CAD build for the part. Positions are in the model's coordinates, mm. A direction names the side the tool comes from. Round coordinates to 2 decimals unless told otherwise and drop trailing zeros. Order: outer loops, then holes, each group sorted by start corner. A loop starts at its lowest first (then second) coordinate and runs counter-clockwise, first axis right, second up. Notation, with made-up numbers: M -37,-32 L -2,-32 A11 ccw -2,-23 Z; hole C 38,-17 d6. An arc over 180 degrees is marked long. Answer as a JSON object with one key per item and string values.
```python
from build123d import *

# Parameters (mm, degrees)
EXTRUDE_1_DEPTH = 1.5
SKETCH_2_R      = 3
EXTRUDE_2_DEPTH = 7
EXTRUDE_START   = 3.5
EXTRUDE_3_DEPTH = 1.5
SKETCH_3_R      = 2.5
EXTRUDE_4_DEPTH = 23
SKETCH_4_R      = 2
EXTRUDE_5_DEPTH = 19.75
CHAMFER_1_SIZE  = 0.39


with BuildPart() as part:
    # Эскиз1 → Бобышка-Вытянуть1 (new body)
    with BuildSketch(Plane.XY):
        Polygon((-4, 2.309401077), (-4, -2.309401077), (0, -4.618802154), (4, -2.309401077), (4, 2.309401077), (0, 4.618802154), align=None)
    extrude(amount=EXTRUDE_1_DEPTH)

    # Эскиз2 → Бобышка-Вытянуть2 (add)
    with BuildSketch(Plane.XY.offset(1.5)):
        Circle(SKETCH_2_R)
    extrude(amount=EXTRUDE_2_DEPTH)

    # Эскиз1<2> → Бобышка-Вытянуть3 (add)
    with BuildSketch(Plane.XY.offset(EXTRUDE_START)):
        Polygon((-4, 2.309401077), (-4, -2.309401077), (0, -4.618802154), (4, -2.309401077), (4, 2.309401077), (0, 4.618802154), align=None)
    extrude(amount=EXTRUDE_3_DEPTH)

    # Эскиз3 → Бобышка-Вытянуть4 (add)
    with BuildSketch(Plane.XY.offset(8.5)):
        Circle(SKETCH_3_R)
    extrude(amount=EXTRUDE_4_DEPTH)

    # Эскиз4 → Бобышка-Вытянуть5 (add)
    with BuildSketch(Plane.XY.offset(31.5)):
        Circle(SKETCH_4_R)
    extrude(amount=EXTRUDE_5_DEPTH)

    # Фаска1
    chamfer_1_edges = [part.edges().sort_by_distance(p)[0] for p in [
        (-2, 0, 51.25),
    ]]
    chamfer(chamfer_1_edges, length=CHAMFER_1_SIZE)


solid = part.part
```
Item 1: Saw through at C-C on z = 41.5. List the corners of the cut face in (x, y).
Worked answers:
{"outline": "C 0,0 d4"}
Item 2: Wall check: line 1 along Z through (x, y) = (-0.5, -2); line 2 along Z through (x, y) = (-3, -1.75); line 3 along Y through (x, z) = (1.5, 27.5). Give the ranges that are in metal, low to high. Write a range as [from, to].
Worked answers:
{"line 1": "z = [0, 31.5]", "line 2": "z = [0, 1.5], [3.5, 5]", "line 3": "y = [-2, 2]"}
Item 3: Drop flat-ended pins along their axis: pin 1 Ø3 at (x, z) = (3, 39.5) entering from -Y; pin 2 Ø1 at (x, z) = (-1, 37.5) entering from +Y; pin 3 Ø4 at (y, z) = (-0.5, 13.5) entering from +X. Give the stop position or say it passes through.
Worked answers:
{"pin 1": "stops at y = -1.32", "pin 2": "stops at y = 1.94", "pin 3": "stops at x = 2.5"}
Item 4: 3-axis set-ups, long thin cutter, end or side, ignore diameter. For faces 1 (the flat face through (1, -3, 3.5)), 2 (the flat face through (-4, 0, 4)), 3 (the cylindrical face through (0, -2, 41)): which of +Z, -Z, +X, -X, +Y, -Y reach the whole face in a straight line?
Worked answers:
{"face 1": "none", "face 2": "+Z, -Z, -X, +Y, -Y", "face 3": "+Z"}
Item 5: Saw through at A-A on y = 0. List the corners of the cut face in (x, z), and give its area (3 significant figures).
Worked answers:
{"outline": "M -4,0 L 4,0 L 4,1.5 L 3,1.5 L 3,3.5 L 4,3.5 L 4,5 L 3,5 L 3,8.5 L 2.5,8.5 L 2.5,31.5 L 2,31.5 L 2,50.86 L 1.61,51.25 L -1.61,51.25 L -2,50.86 L -2,31.5 L -2.5,31.5 L -2.5,8.5 L -3,8.5 L -3,5 L -4,5 L -4,3.5 L -3,3.5 L -3,1.5 L -4,1.5 Z", "area": "251 mm2"}
Item 6: Saw through at B-B on z = 23. List the corners of the cut face in (x, y), and give its area (3 significant figures).
Worked answers:
{"outline": "C 0,0 d5", "area": "19.6 mm2"}
